The model under review builds one solid part; all positions refer to its coordinate system, in mm. Round coordinates to 2 decimals unless told otherwise and drop trailing zeros. Write each loop counter-clockwise with the first axis right and the second up, starting at its lowest first coordinate (ties: lowest second). Pieces come first, ordered by that corner, then holes. Notation, with made-up numbers: (62, -18) -> (86, -18) arc R14 ccw to (86, -1) -> close; hole circle Ø3 at (38.25, 26). An arc over 180 degrees is marked (long way). Return JSON: item names as keys, results as strings. Group by question number.
1. Clearance check with flat-ended pins moving along their axes: P1, Ø5, axis at x = 8, y = 10, coming from the -Z side; P2, Ø1.9, axis at x = -8, y = -10, coming from the -Z side. State where each tip first meets the part, or that it passes through.
2. Take a section at D-D, the plane y = -12.5. Write out the cut boundary in (x, z), then the cut area to 3 significant figures.
3. Mouldability with a two-part tool opening along Y and no side actions: class faces 1 (the flat face through (0, 0, 3)), 2 (the flat face through (0, -15, 1)), 3 (the cylindrical face through (6.73, 9.03, 1.48)) as pulls with the +Y half, pulls with the -Y half, needs draft (parallel to the pull), parting line crosses it, or undercut.
4. Take a section at A-A, the plane z = 1.25. Write out the cut boundary in (x, y).
5. Take a section at C-C, the plane x = 8.5. Write out the cut boundary in (y, z).
6. Take a section at B-B, the plane y = 11.25. Write out the cut boundary in (x, z), then the cut area to 3 significant figures.
7. For line 1 along Y through (x, z) = (8, 2); line 2 along X through (y, z) = (-8.75, 1.9); line 3 along Y through (x, z) = (-9, 0.75), list the stretches that pass through material, from the lowest coordinate up. Write a range as from..to.
from build123d import *

# Parameters (mm, degrees)
ESBO_O1_W                = 26
ESBO_O1_H                = 30
ESBO_O1_R                = 1.6
RESSALTO_EXTRUS_O1_DEPTH = 3
FILETE1_R                = 5


with BuildPart() as part:
    # Esboço1 → Ressalto-extrusão1 (new body)
    with BuildSketch(Plane.XY):
        Rectangle(ESBO_O1_W, ESBO_O1_H)
        with Locations((-8, 10)):
            Circle(ESBO_O1_R, mode=Mode.SUBTRACT)
        with Locations((8, 10)):
            Circle(ESBO_O1_R, mode=Mode.SUBTRACT)
        with Locations((8, -10)):
            Circle(ESBO_O1_R, mode=Mode.SUBTRACT)
        with Locations((-8, -10)):
            Circle(ESBO_O1_R, mode=Mode.SUBTRACT)
    extrude(amount=RESSALTO_EXTRUS_O1_DEPTH)

    # Filete1
    filete1_edges = [part.edges().sort_by_distance(p)[0] for p in [
        (-13, -15, 1.5),
        (-13, 15, 1.5),
        (13, 15, 1.5),
        (13, -15, 1.5),
    ]]
    fillet(filete1_edges, radius=FILETE1_R)


solid = part.part
Output:
{
 "1": {"P1": "stops at z = 0", "P2": "passes through"},
 "2": {"outline": "(-12.33, 0) -> (12.33, 0) -> (12.33, 3) -> (-12.33, 3) -> close", "area": "74.0 mm^2"},
 "3": {"face 1": "needs draft", "face 2": "pulls with the -Y half", "face 3": "undercut"},
 "4": {"outline": "(-13, -10) arc R5 ccw to (-8, -15) -> (8, -15) arc R5 ccw to (13, -10) -> (13, 10) arc R5 ccw to (8, 15) -> (-8, 15) arc R5 ccw to (-13, 10) -> close; hole circle Ø3.2 at (-8, -10); hole circle Ø3.2 at (-8, 10); hole circle Ø3.2 at (8, -10); hole circle Ø3.2 at (8, 10)"},
 "5": {"outline": "(-14.97, 0) -> (-11.52, 0) -> (-11.52, 3) -> (-14.97, 3) -> close; (-8.48, 0) -> (8.48, 0) -> (8.48, 3) -> (-8.48, 3) -> close; (11.52, 0) -> (14.97, 0) -> (14.97, 3) -> (11.52, 3) -> close"},
 "6": {"outline": "(-12.84, 0) -> (-9, 0) -> (-9, 3) -> (-12.84, 3) -> close; (-7, 0) -> (7, 0) -> (7, 3) -> (-7, 3) -> close; (9, 0) -> (12.84, 0) -> (12.84, 3) -> (9, 3) -> close", "area": "65.1 mm^2"},
 "7": {"line 1": "y = -15..-11.6, -8.4..8.4, 11.6..15", "line 2": "x = -13..-9, -7..7, 9..13", "line 3": "y = -14.9..-11.25, -8.75..8.75, 11.25..14.9"}
}
